Input: part model. Units: mm. Frame: model coordinates. A direction names the side the tool comes from. Coordinates: 2 decimals unless noted, no trailing zeros. Write each loop counter-clockwise with the first axis right and the second up, starting at its lowest first coordinate (ties: lowest second). Pieces come first, ordered by that corner, then holes. Notation, with made-up numbers: M 25.25,26 L 56.25,26 A36 ccw 56.25,63 Z; hole C -29.5,1 d6. An arc over 180 degrees is marked long. Use one line per item in the form item = value.
from build123d import *

# Parameters (mm, degrees)
SZKIC1_W                    = 8
SZKIC1_H                    = 8
DODANIE_WYCI_GNI_CIE1_DEPTH = 14
WYTNIJ_WYCI_GNI_CIE1_DEPTH  = 5
SZKIC3_R                    = 1.375
WYTNIJ_WYCI_GNI_CIE2_DEPTH  = 9


with BuildPart() as part:
    # Szkic1 → Dodanie-wyciągnięcie1 (new body)
    with BuildSketch(Plane.XY):
        with Locations((4, 4)):
            Rectangle(SZKIC1_W, SZKIC1_H)
    extrude(amount=DODANIE_WYCI_GNI_CIE1_DEPTH)

    # Szkic2 → Wytnij-wyciągnięcie1 (cut)
    with BuildSketch(Plane(origin=(0, 8, 0), x_dir=(1, 0, 0), z_dir=(0, 1, 0))):
        Polygon((0, -10), (5, -10), (8, -10), (8, -12), (5, -12), (0, -12), align=None)
    extrude(amount=-WYTNIJ_WYCI_GNI_CIE1_DEPTH, mode=Mode.SUBTRACT)

    # Szkic3 → Wytnij-wyciągnięcie2 (cut)
    with BuildSketch(Plane(origin=(0, 0, 0), x_dir=(-1, 0, 0), z_dir=(0, 0, -1))):
        with Locations((-4, 4)):
            Circle(SZKIC3_R)
    extrude(amount=-WYTNIJ_WYCI_GNI_CIE2_DEPTH, mode=Mode.SUBTRACT)


solid = part.part
(1) Set-up query: faces 1 (the cylindrical face through (2.73, 3.47, 4.44)), 2 (the flat face through (0, 4, 7)), 3 (the flat face through (4, 3, 11)). Return all of +Z, -Z, +X, -X, +Y, -Y with unobstructed straight access to the full face (end or side cutting, diameter ignored); none if empty.
Computed:
face_1 = -Z
face_2 = +Z, -Z, -X, +Y, -Y
face_3 = +X, -X, +Y
(2) Section query B-B on x = 4. Return the cut outline in (y, z) (3 decimals), plus the area to 4 significant figures.
Computed:
outline = M 0,0 L 2.625,0 L 2.625,9 L 5.375,9 L 5.375,0 L 8,0 L 8,10 L 3,10 L 3,12 L 8,12 L 8,14 L 0,14 Z
area = 77.25 mm^2
(3) First-contact query: pin 1 Ø1.5 at (x, z) = (6.5, 8) entering from -Y. Flat tip, straight axial feed; report the tip coordinate or a pass-through.
Computed:
pin_1 = 0
(4) Line query: probe 1 along Y at (x, z) = (4, 2.5) (3 decimals); probe 2 along Z at (x, y) = (7, 5.5); probe 3 along Y at (x, z) = (4.5, 1.75). Output: solid intervals per line, ascending.
Computed:
probe_1 = 0 to 2.625, 5.375 to 8
probe_2 = 0 to 10, 12 to 14
probe_3 = 0 to 2.72, 5.28 to 8
(5) Pull-direction query (Z, two-part tool) for faces 4 (the flat face through (4, 6, 12)), 5 (the flat face through (8, 4, 7)), 6 (the flat face through (4, 4, 9)); classes: pulls with the +Z half, pulls with the -Z half, needs draft (parallel to the pull), parting line crosses it, or undercut.
Computed:
face_4 = undercut
face_5 = needs draft
face_6 = pulls with the -Z half
(6) Section query D-D on x = 7.25. Return the cut outline in (y, z).
Computed:
outline = M 0,0 L 8,0 L 8,10 L 3,10 L 3,12 L 8,12 L 8,14 L 0,14 Z
(7) Section query A-A on y = 4. Return the cut outline in (x, z) (3 decimals).
Computed:
outline = M 0,0 L 2.625,0 L 2.625,9 L 5.375,9 L 5.375,0 L 8,0 L 8,10 L 0,10 Z; M 0,12 L 8,12 L 8,14 L 0,14 Z
(8) Section query C-C on z = 3.5. Return the cut outline in (x, y) (3 decimals).
Computed:
outline = M 0,0 L 8,0 L 8,8 L 0,8 Z; hole C 4,4 d2.75
